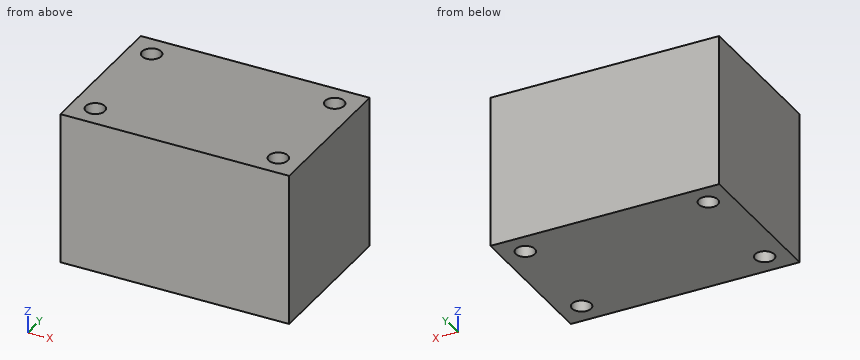
```python
from build123d import *

# Parameters (mm, degrees)
F0_W     = 76.2
F0_H     = 50.8
F1_DEPTH = 25.4
F3_D     = 6.35


with BuildPart() as f1:
    # F0 (on Front) → F1 (new body, symmetric)
    with BuildSketch(Plane.XZ):
        Rectangle(F0_W, F0_H)
    extrude(amount=F1_DEPTH, both=True)

    # F3 (through all)
    with Locations(Plane.XY.offset(25.4)):
        with Locations((30.48, -17.78), (-30.48, -17.78), (30.48, 17.78), (-30.48, 17.78)):
            Hole(F3_D / 2)


solid = f1.part
```
Check sheet for the modelled part. Datum: model origin and axes. Units: mm. Coordinates: 2 decimals unless noted, no trailing zeros. Write each loop counter-clockwise with the first axis right and the second up, starting at its lowest first coordinate (ties: lowest second). Pieces come first, ordered by that corner, then holes. Notation, with made-up numbers: (63.25, 14.5) - (84.25, 14.5) arc R17 cw to (84.25, 45.5) - close; hole circle Ø5 at (55, 19.25). An arc over 180 degrees is marked (long way). One line per question, with ' | ' between items.
Item 1: Sectioned sample at B-B on y = 17.78. Record the boundary of the cut face in (x, z) (3 decimals).
Determined:
outline: (-38.1, -25.4) - (-33.655, -25.4) - (-33.655, 25.4) - (-38.1, 25.4) - close; (-27.305, -25.4) - (27.305, -25.4) - (27.305, 25.4) - (-27.305, 25.4) - close; (33.655, -25.4) - (38.1, -25.4) - (38.1, 25.4) - (33.655, 25.4) - close
Item 2: Thickness scan on line 1 (Y direction, x = -30.48, z = -3) (3 decimals); line 2 (X direction, y = -17.5, z = 13); line 3 (Y direction, x = 31.5, z = 20). Record the ranges inside material, lowest first. Write a range as [from, to].
Determined:
line 1: y = [-25.4, -20.955], [-14.605, 14.605], [20.955, 25.4] | line 2: x = [-38.1, -33.64], [-27.32, 27.32], [33.64, 38.1] | line 3: y = [-25.4, -20.79], [-14.77, 14.77], [20.79, 25.4]
Item 3: Sectioned sample at C-C on x = -30.48. Record the boundary of the cut face in (y, z) (3 decimals), plus the area to 3 significant figures.
Determined:
outline: (-25.4, -25.4) - (-20.955, -25.4) - (-20.955, 25.4) - (-25.4, 25.4) - close; (-14.605, -25.4) - (14.605, -25.4) - (14.605, 25.4) - (-14.605, 25.4) - close; (20.955, -25.4) - (25.4, -25.4) - (25.4, 25.4) - (20.955, 25.4) - close | area: 1,940 mm2
Item 4: Sectioned sample at A-A on z = -18.5. Record the boundary of the cut face in (x, y) (3 decimals).
Determined:
outline: (-38.1, -25.4) - (38.1, -25.4) - (38.1, 25.4) - (-38.1, 25.4) - close; hole circle Ø6.35 at (-30.48, -17.78); hole circle Ø6.35 at (-30.48, 17.78); hole circle Ø6.35 at (30.48, -17.78); hole circle Ø6.35 at (30.48, 17.78)
